Work out the finished part from the listing and answer in its coordinate system (mm). Round coordinates to 2 decimals unless told otherwise and drop trailing zeros. Write each loop counter-clockwise with the first axis right and the second up, starting at its lowest first coordinate (ties: lowest second). Pieces come first, ordered by that corner, then holes. Notation, with made-up numbers: (23, 45.5) -> (73, 45.5) arc R9 ccw to (73, 62.5) -> close; hole circle Ø3 at (36, 22.5). An arc over 180 degrees is marked (long way). One line per item, written item: value.
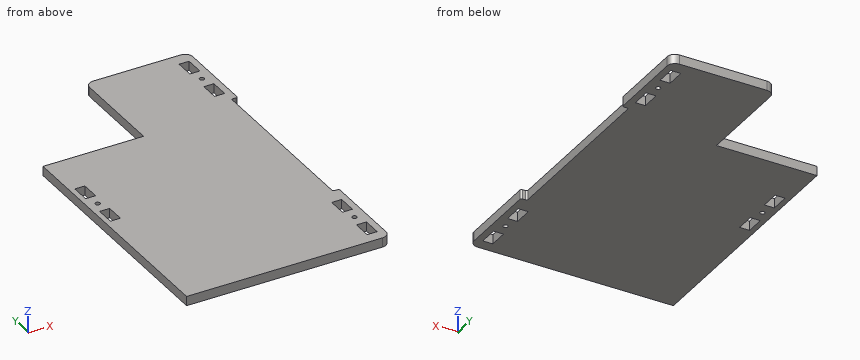
Autodesk Inventor part; units mm, degrees
ref_plane "YZ Plane" through (0, 0, 0) normal (1, 0, 0) x (0, 1, 0)
ref_plane "XZ Plane" through (0, 0, 0) normal (0, 1, 0) x (-1, 0, 0)
ref_plane "XY Plane" through (0, 0, 0) normal (0, 0, 1) x (1, 0, 0)
sketch "Sketch1" plane through (0, 0, 0) normal (0, 0, 1) x (1, 0, 0)
  line L0 (-4.2207, 7.2045) -> (-10.6207, 7.2045)
  line L1 (-10.6207, 7.2045) -> (-10.6207, 19.2045)
  line L2 (-10.6207, 19.2045) -> (-4.2207, 19.2045)
  line L3 (-4.2207, 19.2045) -> (-4.2207, 7.2045)
  circle A0 centre (-7.4207, 27.0045) radius 1.5
  line L4 (-4.2207, 34.8045) -> (-10.6207, 34.8045)
  line L5 (-10.6207, 34.8045) -> (-10.6207, 46.8045)
  line L6 (-10.6207, 46.8045) -> (-4.2207, 46.8045)
  line L7 (-4.2207, 46.8045) -> (-4.2207, 34.8045)
  line L8 (-4.2207, 177.2045) -> (-10.6207, 177.2045)
  line L9 (-10.6207, 177.2045) -> (-10.6207, 189.2045)
  line L10 (-10.6207, 189.2045) -> (-4.2207, 189.2045)
  line L11 (-4.2207, 189.2045) -> (-4.2207, 177.2045)
  circle A1 centre (-7.4207, 197.0045) radius 1.5
  line L12 (-4.2207, 204.8045) -> (-10.6207, 204.8045)
  line L13 (-10.6207, 204.8045) -> (-10.6207, 216.8045)
  line L14 (-10.6207, 216.8045) -> (-4.2207, 216.8045)
  line L15 (-4.2207, 216.8045) -> (-4.2207, 204.8045)
  line L16 (-120.6567, 90.7) -> (-127.0567, 90.7)
  line L17 (-127.0567, 90.7) -> (-127.0567, 102.7)
  line L18 (-127.0567, 102.7) -> (-120.6567, 102.7)
  line L19 (-120.6567, 102.7) -> (-120.6567, 90.7)
  circle A2 centre (-123.8567, 110.5) radius 1.5
  line L20 (-120.6567, 118.3) -> (-127.0567, 118.3)
  line L21 (-127.0567, 118.3) -> (-127.0567, 130.3)
  line L22 (-127.0567, 130.3) -> (-120.6567, 130.3)
  line L23 (-120.6567, 130.3) -> (-120.6567, 118.3)
  line L24 (-66, 160) -> (-130.4, 160)
  line L25 (-130.4, 160) -> (-130.4, 0)
  line L26 (-130.4, 0) -> (-5, 0)
  arc A3 (-5, 0) -> (0, 5) centre (-5, 5) ccw
  line L27 (0, 5) -> (0, 56)
  arc A4 (0, 56) -> (-1, 57) centre (-1, 56) ccw
  line L28 (-1, 57) -> (-3, 57)
  arc A5 (-4, 58) -> (-3, 57) centre (-3, 58) ccw
  line L29 (-4, 58) -> (-4, 169)
  arc A6 (-3, 170) -> (-4, 169) centre (-3, 169) ccw
  line L30 (-3, 170) -> (-1, 170)
  arc A7 (-1, 170) -> (0, 171) centre (-1, 171) ccw
  line L31 (0, 171) -> (0, 220)
  arc A8 (0, 220) -> (-5, 225) centre (-5, 220) ccw
  line L32 (-5, 225) -> (-61, 225)
  arc A9 (-61, 225) -> (-66, 220) centre (-61, 220) ccw
  line L33 (-66, 220) -> (-66, 160)
  point P0 (0, 0)
  point P1 (0, 0)
extrude "Extrusion1" add sketch "Sketch1" along normal blind 6
properties part number "boardCaseBottom"
(1) Find section A-A on y = 14.5. Give the vertices of the cut face in (x, z).
Reported:
outline: (-130.4, 0) -> (-10.62, 0) -> (-10.62, 6) -> (-130.4, 6) -> close; (-4.22, 0) -> (0, 0) -> (0, 6) -> (-4.22, 6) -> close
(2) Find section D-D on z = 0.9. Give the number of separate pieces and of enclosed holes in the cut face, plus the area to 3 significant figures.
Reported:
separate pieces: 1
enclosed holes: 9
area: 24,200 mm2
(3) Flat-ended cylindrical pins translate along their axes: pin 1 Ø3 at (x, z) = (-123, 2) entering from +Y; pin 2 Ø0.6 at (x, z) = (-2, 4) entering from +Y; pin 3 Ø2 at (y, z) = (176.5, 5.5) entering from -X. Find the tip coordinate at first contact, or state that the pin passes through.
Reported:
pin 1: stops at y = 160
pin 2: stops at y = 224.21
pin 3: stops at x = -66
(4) Find section B-B on x = -105. Give the vertices of the cut face in (y, z), plus the area to 3 significant figures.
Reported:
outline: (0, 0) -> (160, 0) -> (160, 6) -> (0, 6) -> close
area: 960 mm2
(5) Consider probe 1 along X at (y, z) = (36.5, 4.7); probe 2 along X at (y, z) = (110.5, 3.7); probe 3 along X at (y, z) = (73.5, 1.5). Determine where each line is inside the solid, lowest interval first.
Reported:
probe 1: x = -130.4 to -10.62, -4.22 to 0
probe 2: x = -130.4 to -125.36, -122.36 to -4
probe 3: x = -130.4 to -4
(6) Find section C-C on y = 114.5. Give the vertices of the cut face in (x, z).
Reported:
outline: (-130.4, 0) -> (-4, 0) -> (-4, 6) -> (-130.4, 6) -> close
